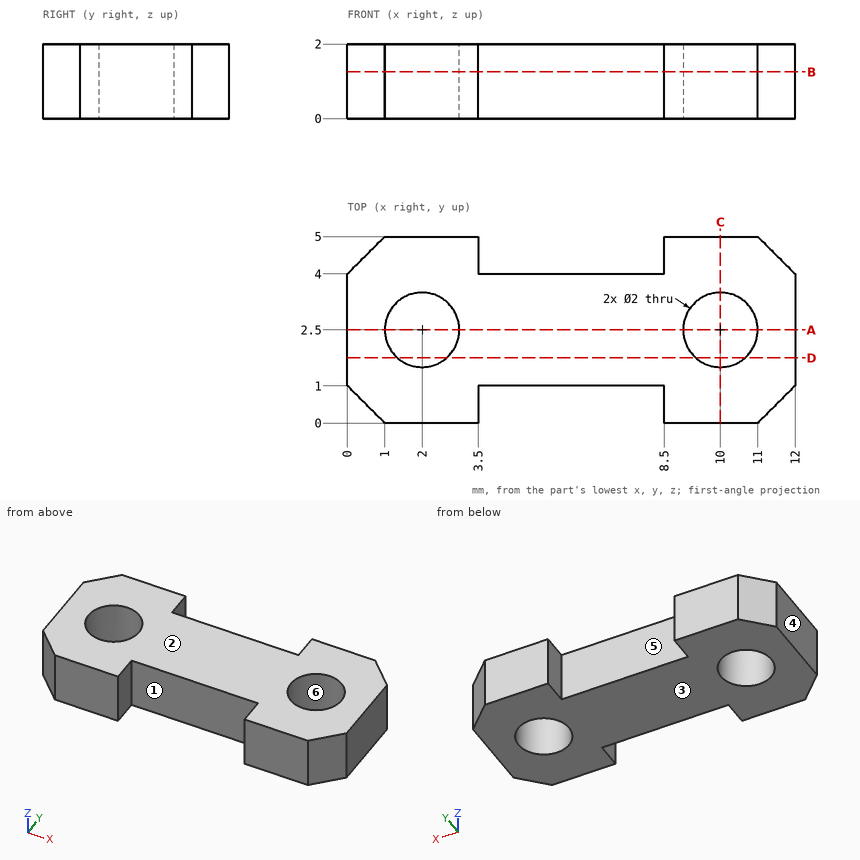
Geometry check sheet. Reference: drawing and pictorial views, mm from the part's lowest x, y, z. A direction names the side the tool comes from. Coordinates: 2 decimals unless noted, no trailing zeros. Write each loop counter-clockwise with the first axis right and the second up, starting at its lowest first coordinate (ties: lowest second). Pieces come first, ordered by that corner, then holes. Notation, with made-up numbers: (24, -5.75) - (82, -5.75) arc R33 ccw to (82, 26.25) - close; hole circle Ø8 at (45.25, 63.5). An arc over 180 degrees is marked (long way). Write item = value, one per line.
Q1. Cross-section at C-C (x = 10). Enter the section's corners in (y, z).
Answer:
outline = (0, 0) - (1.5, 0) - (1.5, 2) - (0, 2) - close; (3.5, 0) - (5, 0) - (5, 2) - (3.5, 2) - close
Q2. Cross-section at B-B (z = 1.25). Enter the section's corners in (x, y), plus the area to 3 significant figures.
Answer:
outline = (0, 1) - (1, 0) - (3.5, 0) - (3.5, 1) - (8.5, 1) - (8.5, 0) - (11, 0) - (12, 1) - (12, 4) - (11, 5) - (8.5, 5) - (8.5, 4) - (3.5, 4) - (3.5, 5) - (1, 5) - (0, 4) - close; hole circle Ø2 at (2, 2.5); hole circle Ø2 at (10, 2.5)
area = 41.7 mm²
Q3. Material ranges on L1, parallel to Y at x = 10, z = 1.5; L2, parallel to Y at x = 4.5, z = 0.4; L3, parallel to X at y = 0.75, z = 1.6, recorded low to high. Write a range as from..to.
Answer:
L1 = 0..1.5, 3.5..5
L2 = 1..4
L3 = 0.25..3.5, 8.5..11.75
Q4. Access from +Z, -Z, +X, -X, +Y, -Y to the whole of each face (thin tool, end or side, straight path). Record for the marked faces 1 and 2.
Answer:
face_1 = +Z, -Z, -Y
face_2 = +Z, +X, -X, +Y, -Y
Q5. Cross-section at D-D (y = 1.75). Enter the section's corners in (x, z).
Answer:
outline = (0, 0) - (1.34, 0) - (1.34, 2) - (0, 2) - close; (2.66, 0) - (9.34, 0) - (9.34, 2) - (2.66, 2) - close; (10.66, 0) - (12, 0) - (12, 2) - (10.66, 2) - close
Q6. Mould release check, pull along X, two halves, no side actions. Record for the marked faces 3, 4, 5 and 6: released by +X, released by -X, zero draft, split by the parting line, or undercut.
Answer:
face_3 = zero draft
face_4 = released by -X
face_5 = undercut
face_6 = undercut
Q7. Go/stop test with flat-tipped pins: pin 1 Ø1 at (x, z) = (6.5, 0.5) entering from +Y; pin 2 Ø1.2 at (x, y) = (10, 2.5) entering from -Z; pin 3 Ø0.8 at (y, z) = (0.5, 1) entering from -X; pin 4 Ø1.1 at (y, z) = (4.5, 0.5) entering from +X. Record where each tip stops, or that it passes through.
Answer:
pin_1 = 4
pin_2 = through
pin_3 = 0.1
pin_4 = 12
Q8. Cross-section at A-A (y = 2.5). Enter the section's corners in (x, z), plus the area to 3 significant figures.
Answer:
outline = (0, 0) - (1, 0) - (1, 2) - (0, 2) - close; (3, 0) - (9, 0) - (9, 2) - (3, 2) - close; (11, 0) - (12, 0) - (12, 2) - (11, 2) - close
area = 16.0 mm²
